```python
from build123d import *

# Parameters (mm, degrees)
IZIM1_W                     = 36.405816339
IZIM1_H                     = 45.737890708
IZIM1_R                     = 2
IZIM1_R_2                   = 2.5
IZIM1_R_3                   = 1.1
Y_KSEKLIK_EKSTR_ZYON3_DEPTH = 5
IZIM2_R                     = 2.5
Y_KSEKLIK_EKSTR_ZYON4_DEPTH = 4
IZIM3_R                     = 1.1
KES_EKSTR_ZYON1_DEPTH       = 17
IZIM5_W                     = 17.110844688
IZIM5_H                     = 73.483837376
Y_KSEKLIK_EKSTR_ZYON6_DEPTH = 14
IZIM6_R                     = 4
KES_EKSTR_ZYON2_DEPTH       = 31


with BuildPart() as part:
    # Çizim1 → Yükseklik-Ekstrüzyon3 (new body)
    # profile 1 of 5: a face of its own
    with BuildSketch(Plane.XY):
        with Locations((0.30959843, 0.881738623)):
            Rectangle(IZIM1_W, IZIM1_H)
        with Locations((-12.59040157, -16.118261377)):
            Circle(IZIM1_R, mode=Mode.SUBTRACT)
        with Locations((13.20959843, -16.118261377)):
            Circle(IZIM1_R, mode=Mode.SUBTRACT)
        with Locations((13.20959843, 17.881738623)):
            Circle(IZIM1_R, mode=Mode.SUBTRACT)
        with Locations((-12.59040157, 17.881738623)):
            Circle(IZIM1_R, mode=Mode.SUBTRACT)
        with Locations((-11.198102854, -6.37596266)):
            Circle(IZIM1_R_2, mode=Mode.SUBTRACT)
        with Locations((9.801897146, -6.37596266)):
            Circle(IZIM1_R_2, mode=Mode.SUBTRACT)
        with Locations((9.801897146, 6.12403734)):
            Circle(IZIM1_R_2, mode=Mode.SUBTRACT)
        with Locations((-11.198102854, 6.12403734)):
            Circle(IZIM1_R_2, mode=Mode.SUBTRACT)
    # profile 2 of 5: a face of its own
    with BuildSketch(Plane.XY):
        with Locations((9.801897146, -6.37596266)):
            Circle(IZIM1_R_2)
        with Locations((9.801897146, -6.37596266)):
            Circle(IZIM1_R_3, mode=Mode.SUBTRACT)
    # profile 3 of 5: a face of its own
    with BuildSketch(Plane.XY):
        with Locations((9.801897146, 6.12403734)):
            Circle(IZIM1_R_2)
        with Locations((9.801897146, 6.12403734)):
            Circle(IZIM1_R_3, mode=Mode.SUBTRACT)
    # profile 4 of 5: a face of its own
    with BuildSketch(Plane.XY):
        with Locations((-11.198102854, 6.12403734)):
            Circle(IZIM1_R_2)
        with Locations((-11.198102854, 6.12403734)):
            Circle(IZIM1_R_3, mode=Mode.SUBTRACT)
    # profile 5 of 5: a face of its own
    with BuildSketch(Plane.XY):
        with Locations((-11.198102854, -6.37596266)):
            Circle(IZIM1_R_2)
        with Locations((-11.198102854, -6.37596266)):
            Circle(IZIM1_R_3, mode=Mode.SUBTRACT)
    extrude(amount=Y_KSEKLIK_EKSTR_ZYON3_DEPTH)

    # Çizim2 → Yükseklik-Ekstrüzyon4 (add)
    with BuildSketch(Plane.XY.offset(5)):
        with Locations((-11.198102854, 6.12403734)):
            Circle(IZIM2_R)
        with Locations((-11.198102854, -6.37596266)):
            Circle(IZIM2_R)
        with Locations((9.801897146, -6.37596266)):
            Circle(IZIM2_R)
        with Locations((9.801897146, 6.12403734)):
            Circle(IZIM2_R)
    extrude(amount=Y_KSEKLIK_EKSTR_ZYON4_DEPTH)

    # Çizim3 → Kes-Ekstrüzyon1 (cut, symmetric)
    with BuildSketch(Plane(origin=(0, 0, 5), x_dir=(-1, 0, 0), z_dir=(0, 0, -1))):
        with Locations(Location((11.198102854, 6.12403734, 0), (0, 0, 180))):
            Circle(IZIM3_R)
        with Locations(Location((11.198102854, -6.37596266, 0), (0, 0, 180))):
            Circle(IZIM3_R)
        with Locations(Location((-9.801897146, -6.37596266, 0), (0, 0, 180))):
            Circle(IZIM3_R)
        with Locations(Location((-9.801897146, 6.12403734, 0), (0, 0, 180))):
            Circle(IZIM3_R)
    extrude(amount=KES_EKSTR_ZYON1_DEPTH, both=True, mode=Mode.SUBTRACT)

    # Çizim5 → Yükseklik-Ekstrüzyon6 (add)
    with BuildSketch(Plane.ZY.offset(17.89330974)):
        Rectangle(IZIM5_W, IZIM5_H)
    extrude(amount=Y_KSEKLIK_EKSTR_ZYON6_DEPTH)

    # Çizim6 → Kes-Ekstrüzyon2 (cut, symmetric)
    with BuildSketch(Plane(origin=(-17.89330974, 0, 0), x_dir=(0, 0, -1), z_dir=(1, 0, 0))):
        with Locations((0, 28)):
            Circle(IZIM6_R)
        with Locations((0, -28)):
            Circle(IZIM6_R)
    extrude(amount=KES_EKSTR_ZYON2_DEPTH, both=True, mode=Mode.SUBTRACT)


solid = part.part
```
Check sheet for the modelled part. Datum: model origin and axes. Units: mm. A direction names the side the tool comes from. Round coordinates to 2 decimals unless told otherwise and drop trailing zeros. Loops run counter-clockwise (first coordinate to the right, second up) from the corner with the lowest first, then second, coordinate; pieces in that order, holes last. Notation, with made-up numbers: (17.25, 44) -> (31.25, 44) arc R15 cw to (31.25, 54) -> close; hole circle Ø8 at (-12.5, 51.25). An arc over 180 degrees is marked (long way). Answer in a Markdown table with one row per item.
Q1. Sectioned sample at B-B on z = 2.75. Give the number of separate pieces and of enclosed holes in the cut face, then the cut area to 3 significant figures.
Data:
| item | result |
|---|---|
| separate pieces | 3 |
| enclosed holes | 8 |
| area | 2,470 mm^2 |
Q2. Go/stop test with flat-tipped pins: P1, Ø1.5, axis at y = -12.5, z = -4, coming from the +X side; P2, Ø2.5, axis at x = -6.5, z = 1.5, coming from the +Y side; P3, Ø8, axis at x = 8, y = 26.5, coming from the +Z side; P4, Ø6.5, axis at y = -28, z = 0, coming from the -X side. Record where each tip stops, or that it passes through.
Data:
| item | result |
|---|---|
| P1 | stops at x = -17.89 |
| P2 | stops at y = 23.75 |
| P3 | stops at z = 5 |
| P4 | passes through |
Q3. Set-up check for faces 1 (the face through (0, 1, 0)), 2 (the face through (7.304, -6.266, 6.972)), 3 (the face through (0, -21.987, 2)): record each of +Z, -Z, +X, -X, +Y, -Y from which the full face is reachable in a straight line by a thin tool's end or side.
Data:
| item | result |
|---|---|
| face 1 | -Z, +X, +Y, -Y |
| face 2 | +Z |
| face 3 | +Z, -Z, +X, -Y |
Q4. Sectioned sample at A-A on y = 28. Enter the section's corners in (x, z).
Data:
| item | result |
|---|---|
| outline | (-31.89, -8.56) -> (-17.89, -8.56) -> (-17.89, -4) -> (-31.89, -4) -> close; (-31.89, 4) -> (-17.89, 4) -> (-17.89, 8.56) -> (-31.89, 8.56) -> close |
Q5. Release check for a two-part mould opening along Z. For faces 4 (the face through (0, 1, 5)), 5 (the face through (-24.795, 31.966, 0.521)), 6 (the face through (-13.18, 4.6, 6.97)) record: released by +Z, released by -Z, zero draft, split by the parting line, or undercut.
Data:
| item | result |
|---|---|
| face 4 | released by +Z |
| face 5 | undercut |
| face 6 | zero draft |
Q6. Thickness scan on L1, parallel to Y at x = -8.5, z = 4.75; L2, parallel to Z at x = -15.5, y = 16.5; L3, parallel to X at y = 30, z = -3.75. Record the ranges inside material, lowest first.
Data:
| item | result |
|---|---|
| L1 | y = -21.99 to 23.75 |
| L2 | z = 0 to 5 |
| L3 | x = -31.89 to -17.89 |
Q7. Sectioned sample at D-D on y = -17. Enter the section's corners in (x, z), then the cut area to 3 significant figures.
Data:
| item | result |
|---|---|
| outline | (-31.89, -8.56) -> (-17.89, -8.56) -> (-17.89, 0) -> (-14.39, 0) -> (-14.39, 5) -> (-17.89, 5) -> (-17.89, 8.56) -> (-31.89, 8.56) -> close; (-10.8, 0) -> (11.41, 0) -> (11.41, 5) -> (-10.8, 5) -> close; (15, 0) -> (18.51, 0) -> (18.51, 5) -> (15, 5) -> close |
| area | 386 mm^2 |
